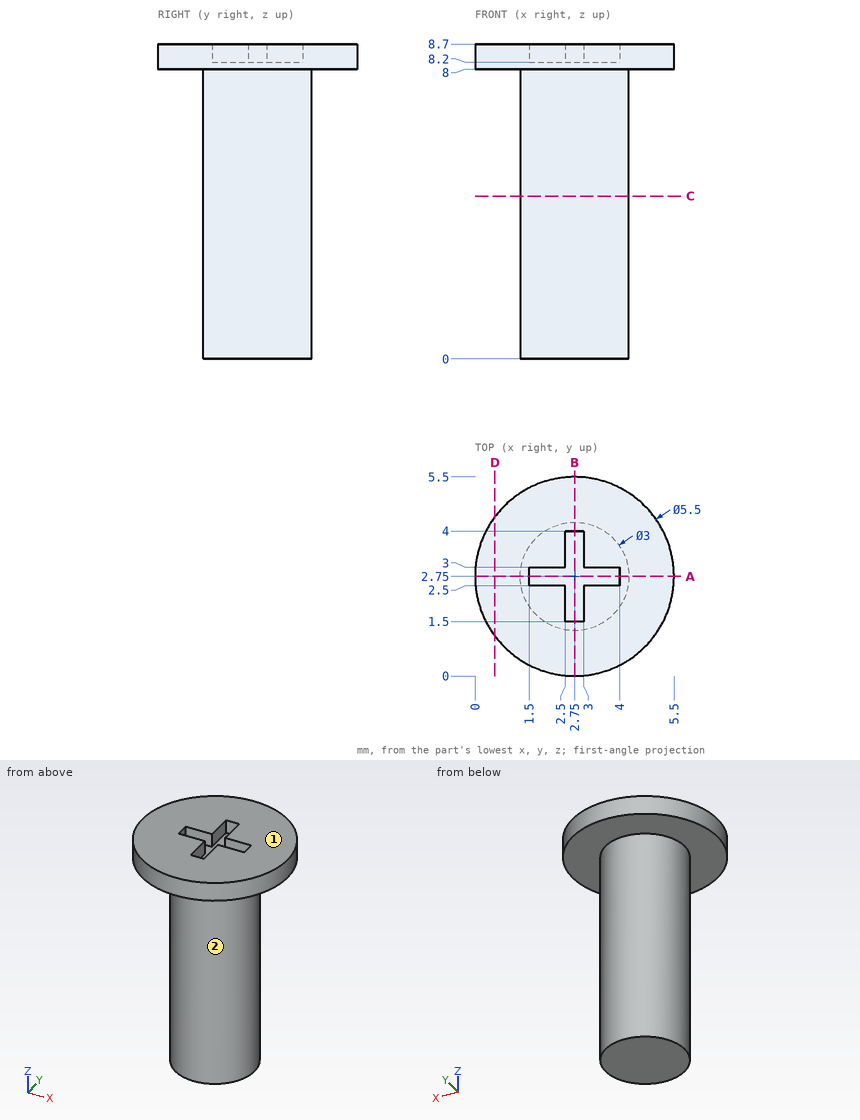
Print and shaded views of the part. All mm, measured from the part's lowest x, y and z. A direction names the side the tool comes from. Round coordinates to 2 decimals unless told otherwise and drop trailing zeros. Order: outer loops, then holes, each group sorted by start corner. A loop starts at its lowest first (then second) coordinate and runs counter-clockwise, first axis right, second up.
Q1. Slice it at D-D (x = 0.55). Write the cut outline in (y, z).
Q2. Which spindle directions (+Z, -Z, +X, -X, +Y, -Y) get a long thin tool onto all of the face, cutting with end or side? Do the marked faces 1 and 2. Say none if no direction does.
Q3. Slice it at C-C (z = 4.5). Write the cut outline in (x, y), and give its area (3 significant figures).
Q4. Wall check: L1, parallel to Z at x = 3.6, y = 4.9; L2, parallel to Z at x = 3.05, y = 2.6; L3, parallel to Y at x = 5.2, z = 8.5. Give the ranges that are in metal, low to high.
Q5. Slice it at A-A (y = 2.75). Write the cut outline in (x, z).
Q6. Drop flat-ended pins along their axis: pin 1 (2 mm diameter, centred on y = 3.5, z = 5, fed in from +X); pin 2 (1 mm diameter, centred on y = 4, z = 2, fed in from +X); pin 3 (0.6 mm diameter, centred on y = 2, z = 8.5, fed in from +X). Give the stop position or say it passes through.
Results below:
1. outline: (1.1, 8) - (4.4, 8) - (4.4, 8.7) - (1.1, 8.7) - close
2. face 1: +Z, +X, -X, +Y, -Y
2. face 2: -Z
3. outline: circle Ø3 at (2.75, 2.75)
3. area: 7.07 mm2
4. L1: z = 8 to 8.7
4. L2: z = 0 to 8.2
4. L3: y = 1.5 to 4
5. outline: (0, 8) - (1.25, 8) - (1.25, 0) - (4.25, 0) - (4.25, 8) - (5.5, 8) - (5.5, 8.7) - (4, 8.7) - (4, 8.2) - (1.5, 8.2) - (1.5, 8.7) - (0, 8.7) - close
6. pin 1: stops at x = 4.25
6. pin 2: stops at x = 4.05
6. pin 3: stops at x = 5.46
